CAD build for the part. Positions are in the model's coordinates, mm. Round coordinates to 2 decimals unless told otherwise and drop trailing zeros. Order: outer loops, then holes, each group sorted by start corner. A loop starts at its lowest first (then second) coordinate and runs counter-clockwise, first axis right, second up. Notation, with made-up numbers: (52, 24) - (89, 24) arc R14 cw to (89, 30) - close; hole circle Ø1 at (68, -5.75). An arc over 180 degrees is marked (long way). Write item = value, one per line.
from build123d import *

# Parameters (mm, degrees)
CROQUIS1_R              = 9
SALIENTE_EXTRUIR1_DEPTH = 1.5
CROQUIS2_R              = 8.5
SALIENTE_EXTRUIR2_DEPTH = 1
VACIADO1_T              = -1
CROQUIS3_R              = 8
CORTAR_EXTRUIR1_DEPTH   = 13.971121771
REDONDEO1_R             = 0.25
REDONDEO3_R             = 0.25
REDONDEO4_R             = 0.25
REDONDEO5_R             = 0.25


with BuildPart() as part:
    # Croquis1 → Saliente-Extruir1 (new body)
    with BuildSketch(Plane(origin=(0, 0, 0), x_dir=(1, 0, 0), z_dir=(0, 1, 0))):
        with Locations(Location((0, 0, 0), (0, 0, 270))):
            Circle(CROQUIS1_R)
    extrude(amount=SALIENTE_EXTRUIR1_DEPTH)

    # Croquis2 → Saliente-Extruir2 (add)
    with BuildSketch(Plane(origin=(0, 1.5, 0), x_dir=(1, 0, 0), z_dir=(0, 1, 0))):
        with Locations(Location((0, 0, 0), (0, 0, 270))):
            Circle(CROQUIS2_R)
    extrude(amount=SALIENTE_EXTRUIR2_DEPTH)

    # Vaciado1
    vaciado1_openings = [part.faces().sort_by_distance(p)[0] for p in [
        (0, 0, 0),
    ]]
    offset(amount=VACIADO1_T, openings=vaciado1_openings, kind=Kind.INTERSECTION)

    # Croquis3 → Cortar-Extruir1 (cut, through all)
    with BuildSketch(Plane(origin=(0, 2.5, 0), x_dir=(1, 0, 0), z_dir=(0, 1, 0))):
        with Locations(Location((0, 0, 0), (0, 0, 270))):
            Circle(CROQUIS3_R)
    extrude(amount=-CORTAR_EXTRUIR1_DEPTH, mode=Mode.SUBTRACT)

    # Redondeo1
    redondeo1_edges = [part.edges().sort_by_distance(p)[0] for p in [
        (0, 1.5, -9),
    ]]
    fillet(redondeo1_edges, radius=REDONDEO1_R)

    # Redondeo3
    redondeo3_edges = [part.edges().sort_by_distance(p)[0] for p in [
        (0, 2.5, -8.5),
    ]]
    fillet(redondeo3_edges, radius=REDONDEO3_R)

    # Redondeo4
    redondeo4_edges = [part.edges().sort_by_distance(p)[0] for p in [
        (0, 0, -9),
    ]]
    fillet(redondeo4_edges, radius=REDONDEO4_R)

    # Redondeo5
    redondeo5_edges = [part.edges().sort_by_distance(p)[0] for p in [
        (0, 0, -8),
    ]]
    fillet(redondeo5_edges, radius=REDONDEO5_R)


solid = part.part
(1) Band-saw the part on A-A on z = 0. List the corners of the cut face in (x, y), plus the area to 3 significant figures.
Solved:
outline = (-9, 0.25) arc R0.25 ccw to (-8.75, 0) - (-8.25, 0) arc R0.25 ccw to (-8, 0.25) - (-8, 2.5) - (-8.25, 2.5) arc R0.25 ccw to (-8.5, 2.25) - (-8.5, 1.5) - (-8.75, 1.5) arc R0.25 ccw to (-9, 1.25) - close; (8, 0.25) arc R0.25 ccw to (8.25, 0) - (8.75, 0) arc R0.25 ccw to (9, 0.25) - (9, 1.25) arc R0.25 ccw to (8.75, 1.5) - (8.5, 1.5) - (8.5, 2.25) arc R0.25 ccw to (8.25, 2.5) - (8, 2.5) - close
area = 3.89 mm²
(2) Drop flat-ended pins along their axis: pin 1 (1.5 mm diameter, centred on y = 2, z = 0.5, fed in from -X); pin 2 (1.5 mm diameter, centred on x = -6, y = 2, fed in from +Z); pin 3 (3 mm diameter, centred on x = 3.5, z = -5, fed in from +Y). Give the stop position or say it passes through.
Solved:
pin_1 = -8.99
pin_2 = 7.02
pin_3 = through
(3) Band-saw the part on B-B on x = 0. List the corners of the cut face in (y, z), plus the area to 3 significant figures.
Solved:
outline = (0, -8.75) arc R0.25 ccw to (0.25, -9) - (1.25, -9) arc R0.25 ccw to (1.5, -8.75) - (1.5, -8.5) - (2.25, -8.5) arc R0.25 ccw to (2.5, -8.25) - (2.5, -8) - (0.25, -8) arc R0.25 ccw to (0, -8.25) - close; (0, 8.25) arc R0.25 ccw to (0.25, 8) - (2.5, 8) - (2.5, 8.25) arc R0.25 ccw to (2.25, 8.5) - (1.5, 8.5) - (1.5, 8.75) arc R0.25 ccw to (1.25, 9) - (0.25, 9) arc R0.25 ccw to (0, 8.75) - close
area = 3.89 mm²
(4) Band-saw the part on D-D on y = 1.8. List the corners of the cut face in (x, z).
Solved:
outline = circle Ø17 at (0, 0); hole circle Ø16 at (0, 0)
(5) Probe line 1 along X through (y, z) = (1.15, 0); line 2 along X through (y, z) = (1.9, 0); line 3 along Z through (x, y) = (-0.5, 1). List the from-to ranges inside material, lowest first.
Solved:
line_1 = -9 to -8, 8 to 9
line_2 = -8.5 to -8, 8 to 8.5
line_3 = -8.99 to -7.98, 7.98 to 8.99
(6) Band-saw the part on C-C on y = 0.7. List the corners of the cut face in (x, z).
Solved:
outline = circle Ø18 at (0, 0); hole circle Ø16 at (0, 0)
(7) Pull direction Z, two halves, no side cores. Call faces 1 (the cylindrical face through (2.703, 0.743, 8.584)), 2 (the flat face through (3, 0, -8)), 3 (the cylindrical face through (-7.81, 1.36, -1.73)): released by +Z, released by -Z, zero draft, split by the parting line, or undercut.
Solved:
face_1 = split by the parting line
face_2 = zero draft
face_3 = undercut
